Work out the finished part from the listing and answer in its coordinate system (mm). A direction names the side the tool comes from. Round coordinates to 2 decimals unless told otherwise and drop trailing zeros. Order: outer loops, then holes, each group sorted by start corner. A loop starts at its lowest first (then second) coordinate and runs counter-clockwise, first axis right, second up. Notation, with made-up numbers: M 78,64 L 109,64 A13 cw 109,84 Z; hole C 77.5,-35.5 d1. An arc over 180 degrees is marked long. Return JSON: item names as keys, results as strings.
from build123d import *

# Parameters (mm, degrees)
SKETCH1_R      = 3.175
EXTRUDE1_DEPTH = 183.769
SKETCH2_R      = 9.525
PISTON_DEPTH   = 2.5


with BuildPart() as part:
    # Sketch1 → Extrude1 (new body)
    with BuildSketch(Plane.XY):
        Circle(SKETCH1_R)
    extrude(amount=EXTRUDE1_DEPTH)

    # Sketch2 → Piston (add, symmetric)
    with BuildSketch(Plane.XY):
        Circle(SKETCH2_R)
    extrude(amount=PISTON_DEPTH, both=True)

    # Sketch3 → Threads (revolve, cut)
    with BuildSketch(Plane(origin=(0, 0, 0), x_dir=(0, 0, -1), z_dir=(1, 0, 0))):
        Polygon((-183.769, 9.525), (-170.569, 9.525), (-170.569, 2.675), (-171.069, 2.675), (-171.069, 3.175), (-183.269, 3.175), (-183.769, 2.675), align=None)
    revolve(axis=Axis((0, 0, 0), (0, 0, 1)), mode=Mode.SUBTRACT)


solid = part.part
Item 1: Each of these flat-tipped pins is pushed along its axis until it touches: pin 1 (5 mm diameter, centred on y = -6, z = 145.5, fed in from -X); pin 2 (4 mm diameter, centred on y = 2, z = 53, fed in from -X) (3 decimals); pin 3 (10 mm diameter, centred on x = 5, z = 20.5, fed in from +Y) (3 decimals); pin 4 (10 mm diameter, centred on x = 7, z = 142, fed in from -Y). Where does it stop, or does it pass through?
Output:
{"pin 1": "passes through", "pin 2": "stops at x = -3.175", "pin 3": "stops at y = 3.175", "pin 4": "stops at y = -2.47"}
Item 2: The mould has two halves that part along Z. Classify faces 4 (the cylindrical face through (-0.69, -3.1, 85.36)), 5 (the flat face through (2, -2, 170.569)), 6 (the flat face through (0, 0, 183.769)): pulls with the +Z half, pulls with the -Z half, needs draft (parallel to the pull), parting line crosses it, or undercut.
Output:
{"face 4": "needs draft", "face 5": "undercut", "face 6": "pulls with the +Z half"}
Item 3: Which of the six approach directions +Z, -Z, +X, -X, +Y, -Y give full straight-line access (tool end or side, diameter ignored) to faces 1 (the cylindrical face through (-7.559, -5.796, 0.035)), 2 (the flat face through (4, 0, 2.5)), 3 (the cylindrical face through (2.61, -0.58, 170.82))?
Output:
{"face 1": "+Z, -Z", "face 2": "+Z", "face 3": "none"}
Item 4: Find section C-C (z = 64.5). Determine the outline of the cut face in (x, y) (3 decimals).
Output:
{"outline": "C 0,0 d6.35"}
Item 5: Find section A-A (y = 0). Determine the outline of the cut face in (x, z) (3 decimals), plus the area to 3 significant figures.
Output:
{"outline": "M -9.525,-2.5 L 9.525,-2.5 L 9.525,2.5 L 3.175,2.5 L 3.175,170.569 L 2.675,170.569 L 2.675,171.069 L 3.175,171.069 L 3.175,183.269 L 2.675,183.769 L -2.675,183.769 L -3.175,183.269 L -3.175,171.069 L -2.675,171.069 L -2.675,170.569 L -3.175,170.569 L -3.175,2.5 L -9.525,2.5 Z", "area": "1,250 mm^2"}
Item 6: Consider line 1 along Z through (x, y) = (-3.5, -5.75); line 2 along X through (y, z) = (0.25, 111). Determine where each line is inside the solid, lowest interval first. Write a range as [from, to].
Output:
{"line 1": "z = [-2.5, 2.5]", "line 2": "x = [-3.17, 3.17]"}
Item 7: Find section D-D (y = 6.75). Determine the outline of the cut face in (x, z), plus the area to 3 significant figures.
Output:
{"outline": "M -6.72,-2.5 L 6.72,-2.5 L 6.72,2.5 L -6.72,2.5 Z", "area": "67.2 mm^2"}
